```python
from build123d import *

# Parameters (mm, degrees)
SKETCH1_W                     = 40
SKETCH1_H                     = 20
BOSS_EXTRUDE1_DEPTH           = 2
SKETCH5_W                     = 50
SKETCH5_H                     = 20
BOSS_EXTRUDE4_DEPTH           = 2
SKETCH6_R                     = 2.35
BOSS_EXTRUDE5_DEPTH           = 4
SKETCH15_R                    = 4.65
CUT_EXTRUDE6_DEPTH            = 6
SKETCH17_W                    = 10
SKETCH17_H                    = 20
CUT_EXTRUDE8_DEPTH            = 43.614551505
CUT_EXTRUDE9_DEPTH            = 2
SKETCH19_R                    = 2.35
BOSS_EXTRUDE6_DEPTH           = 5
BOSS_EXTRUDE7_DEPTH           = 2
SKETCH21_R                    = 5
BOSS_EXTRUDE8_DEPTH           = 10
SKETCH22_R                    = 1
CUT_EXTRUDE10_DEPTH           = 8
CUT_EXTRUDE10_DRAFT           = -1
SKETCH23_W                    = 4
SKETCH23_H                    = 12.6
SKETCH23_H_2                  = 12.600139219
BOSS_EXTRUDE9_DEPTH           = 9
SKETCH24_R                    = 1
CUT_EXTRUDE11_DEPTH           = 6
CUT_EXTRUDE11_DRAFT           = -1
CUT_EXTRUDE11_PROFILE_2_DEPTH = 6
CUT_EXTRUDE11_PROFILE_2_DRAFT = -1
SKETCH25_W                    = 20
SKETCH25_H                    = 2
BOSS_EXTRUDE10_DEPTH          = 4
SKETCH26_W                    = 20
SKETCH26_H                    = 4
BOSS_EXTRUDE11_DEPTH          = 10
FILLET1_R                     = 10
SKETCH27_R                    = 1
CUT_EXTRUDE13_DEPTH           = 49.908077043
SKETCH28_R                    = 2.5
CUT_EXTRUDE14_DEPTH           = 3
BOSS_EXTRUDE12_START          = 1
SKETCH29_R                    = 4.5
SKETCH29_R_2                  = 2.5
BOSS_EXTRUDE12_DEPTH          = 1


with BuildPart() as part:
    # Sketch1 → Boss-Extrude1 (new body)
    with BuildSketch(Plane(origin=(0, 0, 0), x_dir=(1, 0, 0), z_dir=(0, 1, 0))):
        Rectangle(SKETCH1_W, SKETCH1_H)
    extrude(amount=BOSS_EXTRUDE1_DEPTH)

    # Sketch5 → Boss-Extrude4 (add)
    with BuildSketch(Plane(origin=(0, 2, 0), x_dir=(1, 0, 0), z_dir=(0, 1, 0))):
        with Locations((5, 20)):
            Rectangle(SKETCH5_W, SKETCH5_H)
    extrude(amount=-BOSS_EXTRUDE4_DEPTH)

    # Sketch6 → Boss-Extrude5 (add)
    with BuildSketch(Plane(origin=(0, 2, 0), x_dir=(1, 0, 0), z_dir=(0, 1, 0))):
        with Locations(Location((-10, 25, 0), (0, 0, 270))):
            Circle(SKETCH6_R)
        with Locations(Location((10, 25, 0), (0, 0, 270))):
            Circle(SKETCH6_R)
    extrude(amount=BOSS_EXTRUDE5_DEPTH)

    # Sketch15 → Cut-Extrude6 (cut)
    with BuildSketch(Plane(origin=(0, 2, 0), x_dir=(1, 0, 0), z_dir=(0, 1, 0))):
        with Locations(Location((10, 0, 0), (0, 0, 270))):
            Circle(SKETCH15_R)
    extrude(amount=-CUT_EXTRUDE6_DEPTH, mode=Mode.SUBTRACT)

    # Sketch17 → Cut-Extrude8 (cut, through all)
    with BuildSketch(Plane(origin=(0, 2, 0), x_dir=(1, 0, 0), z_dir=(0, 1, 0))):
        with Locations((25, 20)):
            Rectangle(SKETCH17_W, SKETCH17_H)
    extrude(amount=-CUT_EXTRUDE8_DEPTH, mode=Mode.SUBTRACT)

    # Sketch18 → Cut-Extrude9 (cut)
    with BuildSketch(Plane(origin=(0, 2, 0), x_dir=(1, 0, 0), z_dir=(0, 1, 0))):
        Polygon((-11.1, 30), (-20, 10), (-20, 30), align=None)
        Polygon((20, 10), (11.25, 30), (20, 30), align=None)
    extrude(amount=-CUT_EXTRUDE9_DEPTH, mode=Mode.SUBTRACT)

    # Sketch19 → Boss-Extrude6 (add)
    with BuildSketch(Plane(origin=(0, 2, 0), x_dir=(1, 0, 0), z_dir=(0, 1, 0))):
        with Locations(Location((-10, 0, 0), (0, 0, 270))):
            Circle(SKETCH19_R)
    extrude(amount=BOSS_EXTRUDE6_DEPTH)

    # Sketch20 → Boss-Extrude7 (add)
    with BuildSketch(Plane(origin=(0, 2, 0), x_dir=(1, 0, 0), z_dir=(0, 1, 0))):
        Polygon((-20, 10), (-22, 5.505617978), (-22, -12), (-20, -12), (20, -12), (22, -12), (22, 5.428571429), (20, 10), (20, -10), (-20, -10), align=None)
    extrude(amount=-BOSS_EXTRUDE7_DEPTH)

    # Sketch21 → Boss-Extrude8 (add)
    with BuildSketch(Plane(origin=(0, 2, 0), x_dir=(1, 0, 0), z_dir=(0, 1, 0))):
        with Locations(Location((0, 16.787751337, 0), (0, 0, 270))):
            Circle(SKETCH21_R)
    extrude(amount=BOSS_EXTRUDE8_DEPTH)


with BuildPart() as cut_extrude10_tool:
    # Sketch22 → Cut-Extrude10 (with draft: the straight prism first)
    with BuildSketch(Plane(origin=(0, 12, 0), x_dir=(1, 0, 0), z_dir=(0, 1, 0))):
        with Locations((0, 16.787751337)):
            Circle(SKETCH22_R)
    extrude(amount=-CUT_EXTRUDE10_DEPTH)
    # Cut-Extrude10: the draft: its side faces are tilted about the plane it starts from
    cut_extrude10_sides = [cut_extrude10_tool.faces().sort_by_distance(p)[0] for p in [
        (-1, 8, -16.787751337),
    ]]
    draft(cut_extrude10_sides, Plane(origin=(0, 12, 0), x_dir=(1, 0, 0), z_dir=(0, 1, 0)), CUT_EXTRUDE10_DRAFT)


with BuildPart() as part_1:
    add(part.part)

    # Cut-Extrude10: cut by cut_extrude10_tool
    add(cut_extrude10_tool.part, mode=Mode.SUBTRACT)

    # Sketch23 → Boss-Extrude9 (add)
    with BuildSketch(Plane.XZ):
        with Locations((-9.55, 0)):
            Rectangle(SKETCH23_W, SKETCH23_H)
        with Locations((18.549999997, 8.8752e-05)):
            Rectangle(SKETCH23_W, SKETCH23_H_2)
    extrude(amount=BOSS_EXTRUDE9_DEPTH)


with BuildPart() as cut_extrude11_tool:
    # Sketch24 → Cut-Extrude11 (with draft: the straight prism first)
    with BuildSketch(Plane.XZ.offset(9)):
        with Locations((18.267131572, 0.01512814)):
            Circle(SKETCH24_R)
    extrude(amount=-CUT_EXTRUDE11_DEPTH)
    # Cut-Extrude11: the draft: its side faces are tilted about the plane it starts from
    cut_extrude11_sides = [cut_extrude11_tool.faces().sort_by_distance(p)[0] for p in [
        (17.267131572, -6, 0.01512814),
    ]]
    draft(cut_extrude11_sides, Plane.XZ.offset(9), CUT_EXTRUDE11_DRAFT)


with BuildPart() as part_2:
    add(part_1.part)

    # Cut-Extrude11: cut by cut_extrude11_tool
    add(cut_extrude11_tool.part, mode=Mode.SUBTRACT)


with BuildPart() as cut_extrude11_profile_2_tool:
    # Sketch24 → Cut-Extrude11 profile 2 (with draft: the straight prism first)
    with BuildSketch(Plane.XZ.offset(9)):
        with Locations((-9.275, 0)):
            Circle(SKETCH24_R)
    extrude(amount=-CUT_EXTRUDE11_PROFILE_2_DEPTH)
    # Cut-Extrude11 profile 2: the draft: its side faces are tilted about the plane it starts from
    cut_extrude11_profile_2_sides = [cut_extrude11_profile_2_tool.faces().sort_by_distance(p)[0] for p in [
        (-10.275, -6, 0),
    ]]
    draft(cut_extrude11_profile_2_sides, Plane.XZ.offset(9), CUT_EXTRUDE11_PROFILE_2_DRAFT)


with BuildPart() as part_3:
    add(part_2.part)

    # Cut-Extrude11 profile 2: cut by cut_extrude11_profile_2_tool
    add(cut_extrude11_profile_2_tool.part, mode=Mode.SUBTRACT)

    # Sketch25 → Boss-Extrude10 (add)
    with BuildSketch(Plane.XY.offset(12)):
        with Locations((0, 1)):
            Rectangle(SKETCH25_W, SKETCH25_H)
    extrude(amount=BOSS_EXTRUDE10_DEPTH)

    # Sketch26 → Boss-Extrude11 (add)
    with BuildSketch(Plane(origin=(0, 2, 0), x_dir=(1, 0, 0), z_dir=(0, 1, 0))):
        with Locations((0, -14)):
            Rectangle(SKETCH26_W, SKETCH26_H)
    extrude(amount=BOSS_EXTRUDE11_DEPTH)

    # Fillet1
    # the kernel refuses this fillet: 10 mm, written as the material it adds along each edge
    with BuildSketch(Plane(origin=(10, 2, 12), x_dir=(0, 0, 1), z_dir=(0, -1, 0)), Plane(origin=(-10, 0, 12), x_dir=(0, 0, 1), z_dir=(0, 1, 0))) as fillet1_piece_1:
        with BuildLine():
            CenterArc((10, -8), FILLET1_R, 126.869897646, 53.130102354)
            Line((0, -8), (0, 0))
            Line((0, 0), (4, 0))
        make_face()
    extrude(amount=2)

    # Sketch27 → Cut-Extrude13 (cut, through all)
    with BuildSketch(Plane(origin=(0, 0, 12), x_dir=(-1, 0, 0), z_dir=(0, 0, -1))):
        with Locations((0, 7)):
            Circle(SKETCH27_R)
    extrude(amount=-CUT_EXTRUDE13_DEPTH, mode=Mode.SUBTRACT)

    # Sketch28 → Cut-Extrude14 (cut)
    with BuildSketch(Plane.XY.offset(16)):
        with Locations((0, 7)):
            Circle(SKETCH28_R)
    extrude(amount=-CUT_EXTRUDE14_DEPTH, mode=Mode.SUBTRACT)

    # Sketch29 → Boss-Extrude12 (add)
    with BuildSketch(Plane.XY.offset(16).offset(BOSS_EXTRUDE12_START)):
        with Locations((0, 7)):
            Circle(SKETCH29_R)
        with Locations((0, 7)):
            Circle(SKETCH29_R_2, mode=Mode.SUBTRACT)
    extrude(amount=-BOSS_EXTRUDE12_DEPTH)


solid = part_3.part
```
The listing builds one solid part. Answer for the finished solid, in the listing's coordinates (mm). A direction names the side the tool comes from. Coordinates: 2 decimals unless noted, no trailing zeros. Write each loop counter-clockwise with the first axis right and the second up, starting at its lowest first coordinate (ties: lowest second). Pieces come first, ordered by that corner, then holes. Notation, with made-up numbers: (46.25, -3) -> (59.25, -3) arc R4 ccw to (59.25, 2) -> close; hole circle Ø2 at (28.5, -37). An arc over 180 degrees is marked (long way). Write each question's results on one line, items separated by ' | '. Start each with the question number.
1) Straight lines are drawn through the part: probe 1 along X at (y, z) = (-4.5, -2); probe 2 along Y at (x, z) = (0, 15.85); probe 3 along X at (y, z) = (0.5, 0). For each, find the intervals that lie inside material, in ascending order.
2) A cutting plane is placed at B-B (x = -15). Determine the outline of the cut face in (y, z).
3) For a pull along Z with two mould halves and no side action, classify faces 5 (the flat face through (-10.5, -9, 0.1)), 6 (the cylindrical face through (-13.47, 0.986, 13.085)), 7 (the flat face through (-9, -3, 0)) as +Z half, -Z half, draft (parallel to the pull), parting line (faces both ways), or undercut.
4) A cutting plane is placed at A-A (y = -5.25). Determine the outline of the cut face in (x, z) (3 decimals).
5) A tool of negligible diameter and unlimited length cuts with its end or side. For faces 1 (the cylindrical face through (-12.294, 4.465, -0.509)), 2 (the flat face through (10, 6, -25)), 3 (the flat face through (10, 7, 14)), 4 (the flat face through (20.55, -4, 0)), from which of +Z, -Z, +X, -X, +Y, -Y can it reach the whole face along a straight path? Write none if from no direction.
6) Flat-ended cylindrical pins translate along their axes: pin 1 Ø4.5 at (x, y) = (17.5, -5.5) entering from +Z; pin 2 Ø3 at (x, z) = (-16.5, -3) entering from +Y; pin 3 Ø1.6 at (x, y) = (0, 7) entering from -Z. Find the tip coordinate at first contact, or state that the pin passes through.
Values follow:
1) probe 1: -11.55 to -7.55, 16.55 to 20.55 | probe 2: 0 to 4.5, 9.5 to 12 | probe 3: -22 to 5.35, 14.65 to 22
2) outline: (0, -21.24) -> (2, -21.24) -> (2, 12.46) -> (0, 12.46) -> close
3) face 5: draft | face 6: +Z half | face 7: undercut
4) outline: (-11.55, -6.3) -> (-7.55, -6.3) -> (-7.55, 6.3) -> (-11.55, 6.3) -> close; (16.55, -6.3) -> (20.55, -6.3) -> (20.55, 6.3) -> (16.55, 6.3) -> close; hole circle Ø1.869 at (-9.275, 0); hole circle Ø1.869 at (18.267, 0.015)
5) face 1: +Y | face 2: -Z, +X, -X, +Y | face 3: +Z, +X, +Y | face 4: +Z, -Z, +X, -Y
6) pin 1: z = 6.3 | pin 2: y = 2 | pin 3: z = -21.79
